Autodesk Inventor part; units mm, degrees
ref_plane "YZ Plane" through (0, 0, 0) normal (1, 0, 0) x (0, 1, 0)
ref_plane "XZ Plane" through (0, 0, 0) normal (0, 1, 0) x (-1, 0, 0)
ref_plane "XY Plane" through (0, 0, 0) normal (0, 0, 1) x (1, 0, 0)
sketch "Sketch1" plane through (0, 0, 0) normal (0, 1, 0) x (-1, 0, 0)
  line L0 (-12.75, 0) -> (-16.75, 0)
  line L1 (0, 12.75) -> (0, 16.75)
  line L2 (0, -12.75) -> (0, -16.75)
  line L3 (12.75, 0) -> (16.75, 0)
  arc A0 (-12.75, 0) -> (0, -12.75) centre (0, 0) ccw
  arc A1 (12.75, 0) -> (0, 12.75) centre (0, 0) ccw
  arc A2 (-16.75, 0) -> (0, -16.75) centre (0, 0) ccw
  arc A3 (16.75, 0) -> (0, 16.75) centre (0, 0) ccw
extrude "Extrusion1" add sketch "Sketch1" along normal blind 3
sketch "Sketch2" plane through (0, 0, 0) normal (0, -1, 0) x (1, 0, 0)
  circle A0 centre (0, 0) radius 16.75
  arc A1 (0, -16.75) -> (16.75, 0) centre (0, 0) ccw
  circle A2 centre (0, 0) radius 20.75
  arc A3 (0, -16.75) -> (16.75, 0) centre (0, 0) ccw
  dimension "d4" = 4
  dimension "d5" = 33.5
extrude "Extrusion2" add sketch "Sketch2" against normal blind 8
sketch "Sketch3" plane through (0, 0, 0) normal (1, 0, 0) x (0, 1, 0)
  line L0 (8, -20.75) -> (8, 20.75)
  line L1 (8, 16.75) -> (8, -16.75)
  line L2 (8, 16.75) -> (8, -16.75)
  line L3 (8, -16.75) -> (13, -16.75)
  line L4 (13, -16.75) -> (21, -6.75)
  line L5 (8, -20.75) -> (8, 20.75)
  line L6 (3, 0) -> (3, -12.75)
  line L7 (0, -12.75) -> (3, -12.75)
  line L8 (21, -6.75) -> (21, -4.75)
  line L9 (21.5, -4.75) -> (21.5, -6.8032)
  line L10 (14.9225, -20.75) -> (8, -20.75)
  line L11 (14.9225, -20.75) -> (21.5, -6.8032)
  line L12 (8, -16.75) -> (8, -20.75)
  line L13 (21, -4.75) -> (21.5, -4.75)
  line L14 (-4.3, 0) -> (25.8, 0)
  point P0 (0, 0)
  dimension "d8" = 5
  dimension "d9" = 8
  dimension "d10" = 6
  dimension "d11" = 2
  dimension "d12" = 0.5
revolve "Revolution1" add sketch "Sketch3" angle 360 about axis through (0, -10, 0) along (0, 1, 0)
properties part number "Parte superior"
Geometry: final body of the model. Coordinates: model frame, mm. A direction names the side the tool comes from. Round coordinates to 2 decimals unless told otherwise and drop trailing zeros. Write each loop counter-clockwise with the first axis right and the second up, starting at its lowest first coordinate (ties: lowest second). Pieces come first, ordered by that corner, then holes.
Item 1: Pin query (flat end, axial travel): P1, Ø1.5, axis at y = 1.5, z = 14.5, coming from the +X side; P2, Ø3.5, axis at x = -14.5, y = 1.5, coming from the -Z side; P3, Ø0.9, axis at y = 1.5, z = -15, coming from the -X side. Return the tip coordinate at first contact, or that it passes through.
Item 2: Section query B-B (y = 5). Return loops of the section in (x, z).
Item 3: Material intervals for L1, parallel to Z at x = 0, y = 5.5; L2, parallel to X at y = 4.75, z = 15, sorted ascending.
Item 4: Set-up query: faces 1 (the face through (-10, 0, 10)), 2 (the face through (9, 3, -10)), 3 (the face through (0, 1, -15)). Return all of +Z, -Z, +X, -X, +Y, -Y with unobstructed straight access to the full face (end or side cutting, diameter ignored); none if empty.
Item 5: Mould query, pull axis Z, two halves, no side actions, for faces 4 (the face through (2.3, 21.1, -7.3)), 5 (the face through (-5, 21.5, -1)), 6 (the face through (-15, 1, 0)). Classes: +Z half, -Z half, draft (parallel to the pull), parting line (faces both ways), or undercut.
Item 6: Section query A-A (y = 2). Return loops of the section in (x, z), plus the area to 3 significant figures.
Completed:
1. P1: stops at x = 15.54
1. P2: stops at z = -16.37
1. P3: stops at x = -14.79
2. outline: circle Ø41.5 at (0, 0); hole circle Ø33.5 at (0, 0)
3. L1: z = -20.75 to -16.75, 16.75 to 20.75
3. L2: x = -14.34 to -7.45, 7.45 to 14.34
4. face 1: +Z, -Z, +X, -X, -Y
4. face 2: none
4. face 3: -Y
5. face 4: parting line
5. face 5: draft
5. face 6: undercut
6. outline: circle Ø41.5 at (0, 0); hole (-16.75, 0) arc R16.75 ccw to (0, -16.75) - (0, -12.75) arc R12.75 ccw to (12.75, 0) - (16.75, 0) arc R16.75 ccw to (0, 16.75) - (0, 12.75) arc R12.75 ccw to (-12.75, 0) - close
6. area: 657 mm2
